For this review, take the finished solid that the model builds, in its own axes (mm). Face numbers are marked on the shaded views. Coordinates: 2 decimals unless noted, no trailing zeros. Write each loop counter-clockwise with the first axis right and the second up, starting at its lowest first coordinate (ties: lowest second). Pieces come first, ordered by that corner, then holes. Notation, with made-up numbers: M 0,16.5 L 31,16.5 A22 cw 31,39.5 Z; hole C -3.75,66.5 d2. An arc over 180 degrees is marked long. One line per question, with ' | ' between items.
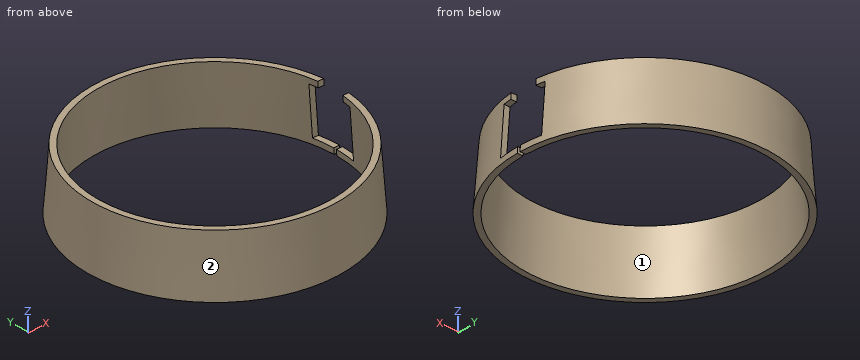
from build123d import *

# Parameters (mm, degrees)
BOX013_W     = 30
BOX013_H     = 9.3
BOX013_DEPTH = 25.5
BOX012_W     = 30
BOX012_H     = 15.3
BOX012_DEPTH = 16.5
BOX014_W     = 30
BOX014_H     = 1
BOX014_DEPTH = 25.5


with BuildPart() as cube013:
    # Box013 → Box013 (new body)
    with BuildSketch(Plane(origin=(24, -4.65, 2), x_dir=(1, 0, 0), z_dir=(0, 0, 1))):
        with Locations((15, 4.65)):
            Rectangle(BOX013_W, BOX013_H)
    extrude(amount=BOX013_DEPTH)


with BuildPart() as cube012:
    # Box012 → Box012 (new body)
    with BuildSketch(Plane(origin=(24, -7.65, 2), x_dir=(1, 0, 0), z_dir=(0, 0, 1))):
        with Locations((15, 7.65)):
            Rectangle(BOX012_W, BOX012_H)
    extrude(amount=BOX012_DEPTH)


with BuildPart() as obj1:
    # Box014 → Box014 (new body)
    with BuildSketch(Plane(origin=(24, -0.5, -2), x_dir=(1, 0, 0), z_dir=(0, 0, 1))):
        with Locations((15, 0.5)):
            Rectangle(BOX014_W, BOX014_H)
    extrude(amount=BOX014_DEPTH)

    # Fusion006: union Cube013, Cube012
    add(cube013.part)
    add(cube012.part)


with BuildPart() as cone_chico:
    # Cone → Cone (revolve)
    with BuildSketch(Plane.XZ):
        Polygon((0, 0), (41.5, 0), (40, 20.5), (0, 20.5), align=None)
    revolve(axis=Axis((0, 0, 0), (0, 0, 1)))


with BuildPart() as obj2:
    # Cone001 → Cone001 (revolve)
    with BuildSketch(Plane.XZ):
        Polygon((0, 0), (43.5, 0), (42, 20.5), (0, 20.5), align=None)
    revolve(axis=Axis((0, 0, 0), (0, 0, 1)))

    # Cut015014: cut Cone_chico
    add(cone_chico.part, mode=Mode.SUBTRACT)

    # Cut015027: cut obj1
    add(obj1.part, mode=Mode.SUBTRACT)


solid = obj2.part
1) The part is to be moulded in two halves that separate along X. For the marked faces 1 and 2, say which applies: +X half, -X half, draft (parallel to the pull), parting line (faces both ways), or undercut.
Responses:
face 1: undercut | face 2: parting line
2) We need section C-C on z = 14. State the section outline as (x, y) points.
Responses:
outline: M 39.75,-7.65 A40.48 cw long 39.75,7.65 L 41.78,7.65 A42.48 ccw long 41.78,-7.65 Z
3) We need section A-A on y = -6. State how many separate pieces and enclosed holes the cut face has, then the cut area to 3 significant figures.
Responses:
separate pieces: 3 | enclosed holes: 0 | area: 49.5 mm^2
4) We need section B-B on z = 8. State the section outline as (x, y) points.
Responses:
outline: M 40.19,-7.65 A40.91 cw long 40.19,7.65 L 42.23,7.65 A42.91 ccw long 42.23,-7.65 Z
5) Insertion check: pin 1 Ø4 at (x, z) = (15, 10) entering from +Y; pin 2 Ø6 at (x, z) = (-23.5, 17) entering from +Y; pin 3 Ø3 at (x, y) = (41.5, 2.5) entering from +Z. Each pin has a flat end and moves straight along its axis. Give the tip position at first contact, or say it passes through.
Responses:
pin 1: y = 40.76 | pin 2: y = 36.97 | pin 3: z = 2
6) To check wall thickness, follow line 1 along Y through (x, z) = (27, 9.75); line 2 along Y through (x, z) = (-38, 5.75); line 3 along X through (y, z) = (25.5, 14.75). State the ranges of each line that lie inside material, in increasing order. Write a range as [from, to].
Responses:
line 1: [-33.19, -30.57], [30.57, 33.19] | line 2: [-20.29, -15.6], [15.6, 20.29] | line 3: [-33.9, -31.36], [31.36, 33.9]
